Autodesk Inventor part; units mm, degrees
ref_plane "YZ Plane" through (0, 0, 0) normal (1, 0, 0) x (0, 1, 0)
ref_plane "XZ Plane" through (0, 0, 0) normal (0, 1, 0) x (-1, 0, 0)
ref_plane "XY Plane" through (0, 0, 0) normal (0, 0, 1) x (1, 0, 0)
sketch "Sketch1" plane through (0, 0, 0) normal (0, 0, 1) x (1, 0, 0)
  line L0 (-5, 20) -> (-5, 9.1421)
  line L1 (0, 10) -> (0, 17.0552) construction
  line L2 (5, 20) -> (5, 9.1421)
  line L3 (5, 10) -> (-5, 10) construction
  line L4 (0, 10) -> (0, 20) construction
  line L5 (-1.5, 20) -> (-1.5, 10)
  line L6 (1.5, 20) -> (1.5, 10)
  line L7 (5, 20) -> (1.5, 20)
  line L8 (-1.5, 20) -> (-5, 20)
  line L9 (-1.5, 10) -> (1.5, 10)
  arc A0 (-5, 9.1421) -> (5, 9.1421) centre (0, -5) ccw
  circle A1 centre (0, -5) radius 12.5
  dimension "d46" = 1.5
  dimension "d61" = 25
extrude "Extrusion1" add sketch "Sketch1" along normal blind 5
sketch "Sketch4" plane through (5, 5.9087, 0) normal (1, 0, 0) x (0, 0, -1)
  line L0 (0, 14.0913) -> (-5, 14.0913) construction
  line L1 (-2.5, 14.0913) -> (-2.5, 9.0913) construction
  circle A0 centre (-2.5, 9.0913) radius 1.5
  point P0 (0, -5.9087)
  dimension "d30" = 5
  dimension "d31" = 3
extrude "Extrusion4" cut sketch "Sketch4" against normal blind 10
ref_plane "Work Plane1" through (0, 5.9087, 0) normal (1, 0, 0) x (0, 0, -1)
ref_plane "Work Plane2" through (0, 5.9087, 0) normal (1, 0, 0) x (0, 0, -1)
sketch "Sketch14" plane through (0, 5.9087, 0) normal (1, 0, 0) x (0, 0, -1)
  line L0 (-5, 1.5913) -> (-20, 1.5913)
  line L1 (-20, 1.5913) -> (-20, 4.0913)
  line L2 (-20, 4.0913) -> (-5, 4.0913)
  line L3 (-5, 1.5913) -> (-5, -23.4087) construction
  line L4 (-5, -10.9087) -> (-20, -10.9087) construction
  line L5 (-5, -23.4087) -> (-5, 1.5913)
  line L6 (-5, 4.0913) -> (-5, 1.5913)
  point P0 (0, -5.9087)
  dimension "d62" = 15
  dimension "d63" = 2.5
  dimension "d64" = 15
revolve "Revolution3" add sketch "Sketch14" angle 360 about axis through (0, -5, 5) along (0, 0, 1)
sketch "Sketch15" plane through (0, 5.9087, 0) normal (1, 0, 0) x (0, 0, -1)
  line L0 (-20, -23.4087) -> (-20, 1.5913)
  arc A0 (-20, 1.5913) -> (-32.5, -10.9087) centre (-20, -10.9087) ccw
  arc A1 (-20, 4.0913) -> (-35, -10.9087) centre (-20, -10.9087) ccw
  line L1 (-32.5, -10.9087) -> (-35, -10.9087) construction
  line L2 (-20, 1.5913) -> (-20, -23.4087) construction
  line L3 (-20, -25.9087) -> (-20, 4.0913)
  line L4 (-20, 1.5913) -> (-20, 4.0913)
  line L5 (-32.5, -10.9087) -> (-35, -10.9087)
  point P0 (0, -5.9087)
  dimension "d67" = 30
revolve "Revolution4" add sketch "Sketch15" angle 360 about axis through (0, -5, 32.5) along (0, 0, 1)
properties part number "beta_dummy _thumb"
Work out the finished part from the listing and answer in its coordinate system (mm). A direction names the side the tool comes from. Coordinates: 2 decimals unless noted, no trailing zeros. Write each loop counter-clockwise with the first axis right and the second up, starting at its lowest first coordinate (ties: lowest second). Pieces come first, ordered by that corner, then holes. Notation, with made-up numbers: M -27,-38.75 L 0,-38.75 A24 cw 0,-12.75 Z; hole C -14.75,62.25 d4. An arc over 180 degrees is marked long. Use one line per item in the form item = value. Start each with the question number.
1. Straight lines are drawn through the part: probe 1 along Y at (x, z) = (0, 8.5); probe 2 along Y at (x, z) = (-4.15, 2.5); probe 3 along X at (y, z) = (-5, 2). For each, find the intervals that lie inside material, in ascending order. Write a range as from..to.
2. The part is cut by section B-B (y = 15). Give the vertices of the cut face in (x, z).
3. The part is cut by section C-C (z = 6). Give the vertices of the cut face in (x, y).
4. Each of these flat-tipped pins is pushed along its axis until it touches: P1, Ø2, axis at x = 4.5, z = 21.5, coming from the -Y side; P2, Ø2.5, axis at x = -1.5, y = 15.5, coming from the +Z side; P3, Ø0.9, axis at x = -0.5, z = 1.5, coming from the +Y side; P4, Ø1.8, axis at y = 15, z = 2.5, coming from the +X side. Where does it stop, or does it pass through?
5. The part is cut by section A-A (z = 2.5). Give the vertices of the cut face in (x, y).
6. The mould has two halves that part along Z. Classify faces 1 (the face through (1.5, 16, 1)), 2 (the face through (4, 15, 5)), 3 (the face through (-3.226, 14.425, 1.114)): released by +Z, released by -Z, zero draft, split by the parting line, or undercut.
7. A tool of negligible diameter and unlimited length cuts with its end or side. For faces 4 (the face through (5, 13, 2)), 5 (the face through (-5, 13, 2)), 6 (the face through (0, 10, 2)), from which of +Z, -Z, +X, -X, +Y, -Y can it reach the whole face along a straight path? Write none if from no direction.
Evaluation:
q1.probe_1 = -20..-17.5, 7.5..10
q1.probe_2 = -19.41..-16.79, 6.79..13.5, 16.5..20
q1.probe_3 = -15..-12.5, 12.5..15
q2.outline = M -5,0 L -1.5,0 L -1.5,1 L -5,1 Z; M -5,4 L -1.5,4 L -1.5,5 L -5,5 Z; M 1.5,0 L 5,0 L 5,1 L 1.5,1 Z; M 1.5,4 L 5,4 L 5,5 L 1.5,5 Z
q3.outline = C 0,-5 d30; hole C 0,-5 d25
q4.P1 = -19.53
q4.P2 = 5
q4.P3 = 10
q4.P4 = through
q5.outline = M -5,9.14 A15 ccw long 5,9.14 L 5,13.5 L 1.5,13.5 L 1.5,10 L -1.5,10 L -1.5,13.5 L -5,13.5 Z; M -5,16.5 L -1.5,16.5 L -1.5,20 L -5,20 Z; M 1.5,16.5 L 5,16.5 L 5,20 L 1.5,20 Z; hole C 0,-5 d25
q6.face_1 = zero draft
q6.face_2 = released by +Z
q6.face_3 = undercut
q7.face_4 = +Z, -Z, +X, +Y
q7.face_5 = +Z, -Z, -X, +Y
q7.face_6 = +Z, -Z, +Y
